Geometry: see drawing. Coordinates: mm, zero at the bounding-box minimum. Coordinates: 2 decimals unless noted, no trailing zeros. Order: outer loops, then holes, each group sorted by start corner. A loop starts at its lowest first (then second) coordinate and runs counter-clockwise, first axis right, second up. Notation, with made-up numbers: M 77,72 L 101,72 A16 cw 101,94 Z; hole C 12,-22.75 d5. An arc over 180 degrees is marked long. One line per item, written item: value.
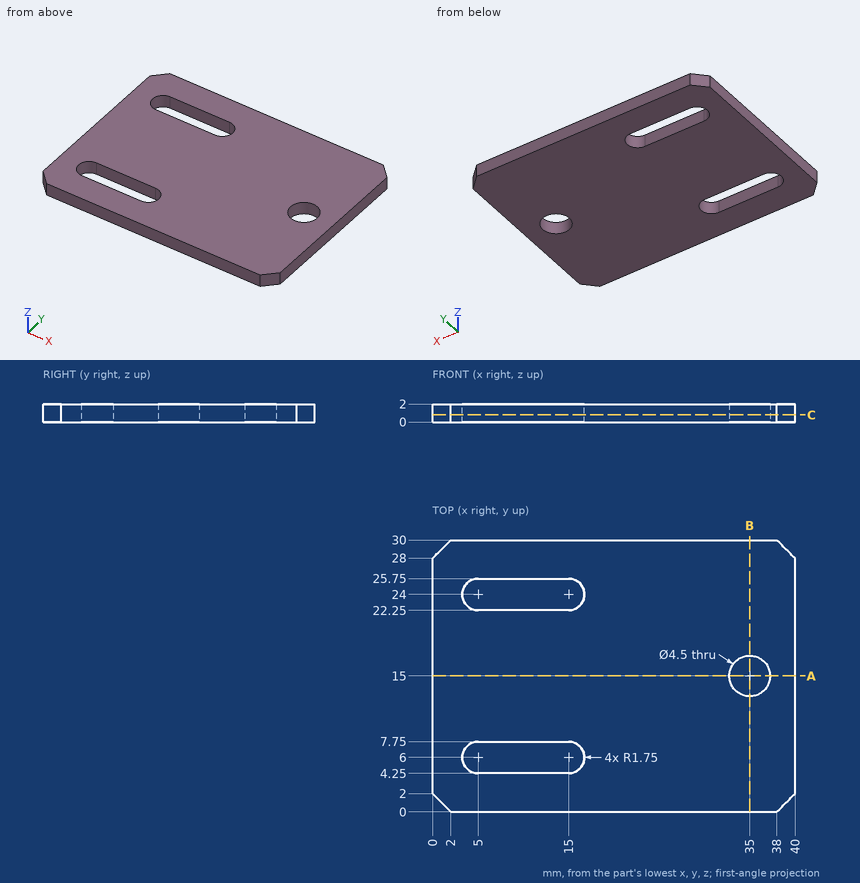
(1) Cut plane B-B on x = 35. Output: boundary loops of the cut face in (y, z).
Data:
outline: M 0,0 L 12.75,0 L 12.75,2 L 0,2 Z; M 17.25,0 L 30,0 L 30,2 L 17.25,2 Z
(2) First-contact query: pin 1 (5 mm diameter, centred on x = 17.5, y = 8.5, fed in from -Z). Flat tip, straight axial feed; report the tip coordinate or a pass-through.
Data:
pin 1: stops at z = 0
(3) Cut plane C-C on z = 0.8. Output: boundary loops of the cut face in (x, y).
Data:
outline: M 0,2 L 2,0 L 38,0 L 40,2 L 40,28 L 38,30 L 2,30 L 0,28 Z; hole M 5,4.25 L 15,4.25 A1.75 ccw 15,7.75 L 5,7.75 A1.75 ccw Z; hole M 5,22.25 L 15,22.25 A1.75 ccw 15,25.75 L 5,25.75 A1.75 ccw Z; hole C 35,15 d4.5
(4) Ray query, line 1 (Y direction, x = 9, z = 1.75); line 2 (Y direction, x = 35, z = 0.9). Return the intervals inside material, ascending. Write a range as from..to.
Data:
line 1: y = 0..4.25, 7.75..22.25, 25.75..30
line 2: y = 0..12.75, 17.25..30
(5) Cut plane A-A on y = 15. Output: boundary loops of the cut face in (x, z), plus the area to 3 significant figures.
Data:
outline: M 0,0 L 32.75,0 L 32.75,2 L 0,2 Z; M 37.25,0 L 40,0 L 40,2 L 37.25,2 Z
area: 71.0 mm2
